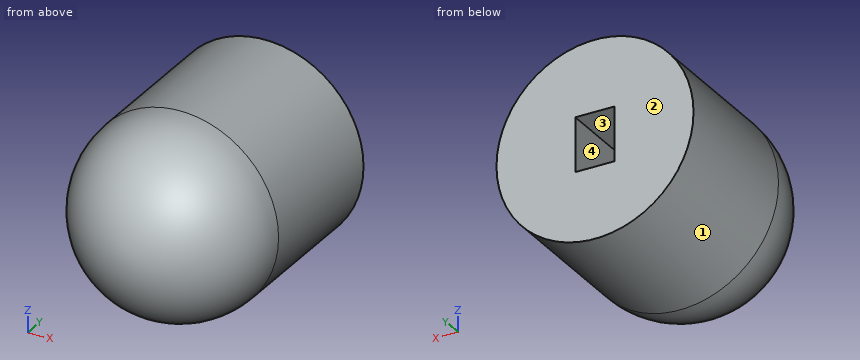
Autodesk Inventor part; units mm, degrees
ref_plane "YZ Plane" through (0, 0, 0) normal (1, 0, 0) x (0, 1, 0)
ref_plane "XZ Plane" through (0, 0, 0) normal (0, 1, 0) x (-1, 0, 0)
ref_plane "XY Plane" through (0, 0, 0) normal (0, 0, 1) x (1, 0, 0)
sketch "Sketch1" plane through (0, 0, 0) normal (0, 1, 0) x (-1, 0, 0)
  line L0 (-0.8, 1.1) -> (0.8, 1.1)
  line L1 (0.8, 1.1) -> (0.8, -1.1)
  line L2 (0.8, -1.1) -> (-0.8, -1.1)
  line L3 (-0.8, -1.1) -> (-0.8, 1.1)
  line L4 (-0.8, 1.1) -> (0.8, -1.1) construction
  line L5 (0.8, 1.1) -> (-0.8, -1.1) construction
  circle A0 centre (0, 0) radius 4
  dimension "d0" = 1.6
  dimension "d1" = 2.2
  dimension "d2" = 8
extrude "Extrusion1" add sketch "Sketch1" along normal blind 10
extrude "Extrusion2" add sketch "Sketch1" along normal blind 5 contours L0 L1 L2 L3
fillet "Fillet1" radius 4 1 edges at (4, 0, 0)
properties part number "Joy"
Verification items for the finished model (mm, model axes). Face numbers are marked on the shaded views. Round coordinates to 2 decimals unless told otherwise and drop trailing zeros. Loops run counter-clockwise (first coordinate to the right, second up) from the corner with the lowest first, then second, coordinate; pieces in that order, holes last. Notation, with made-up numbers: (11.5, 0.25) - (36.5, 0.25) arc R15 cw to (36.5, 20.25) - close; hole circle Ø3 at (41.5, 47). An arc over 180 degrees is marked (long way). Use one line per item in the form item = value.
1. Section check D-D on y = 4.5. Record the cut outline in (x, z), and give its area (3 significant figures).
A:
outline = circle Ø8 at (0, 0)
area = 50.3 mm²
2. Section check C-C on x = 0. Record the cut outline in (y, z).
A:
outline = (4, -4) - (10, -4) - (10, -1.1) - (5, -1.1) - (5, 1.1) - (10, 1.1) - (10, 4) - (4, 4) arc R4 ccw to start
3. Scan lines: probe 1 along Z at (x, y) = (0, 9.25); probe 2 along X at (y, z) = (7.25, 0.5); probe 3 along Z at (x, y) = (3, 4.5). Record each from-to range of solid material in increasing order.
A:
probe_1 = -4 to -1.1, 1.1 to 4
probe_2 = -3.97 to -0.8, 0.8 to 3.97
probe_3 = -2.65 to 2.65
4. Draft check along X on the marked faces 1, 2, 3 and 4. Enter one of: pulls with the +X half, pulls with the -X half, needs draft (parallel to the pull), parting line crosses it, or undercut.
A:
face_1 = parting line crosses it
face_2 = needs draft
face_3 = undercut
face_4 = undercut
5. Section check B-B on z = 0. Record the cut outline in (x, y), and give its area (3 significant figures).
A:
outline = (-4, 4) arc R4 ccw to (4, 4) - (4, 10) - (0.8, 10) - (0.8, 5) - (-0.8, 5) - (-0.8, 10) - (-4, 10) - close
area = 65.1 mm²
6. Gauge pin test, flat ends, axial feed: pin 1 Ø1.5 at (x, y) = (-1, 4) entering from -Z; pin 2 Ø3 at (x, z) = (0, -1) entering from -Y; pin 3 Ø1 at (x, y) = (2.5, 6) entering from +Z; pin 4 Ø0.7 at (y, z) = (6.5, 0.5) entering from +X. Record the tip position at first contact, or that the pin passes through.
A:
pin_1 = -3.99
pin_2 = 0
pin_3 = 3.46
pin_4 = 4
7. Section check A-A on y = 6.5. Record the cut outline in (x, z), and give its area (3 significant figures).
A:
outline = circle Ø8 at (0, 0); hole (-0.8, -1.1) - (0.8, -1.1) - (0.8, 1.1) - (-0.8, 1.1) - close
area = 46.7 mm²
